Part model, mm, in its own coordinate system. Round coordinates to 2 decimals unless told otherwise and drop trailing zeros. Loops run counter-clockwise (first coordinate to the right, second up) from the corner with the lowest first, then second, coordinate; pieces in that order, holes last.
1) Band-saw the part on C-C, the plane z = 75. Write the cut outline in (x, y).
2) Band-saw the part on B-B, the plane x = -38.5. Write the cut outline in (y, z).
3) Band-saw the part on D-D, the plane x = -32. State how many separate pieces and enclosed holes the cut face has, then the cut area to 3 significant figures.
4) Band-saw the part on A-A, the plane z = 65. Write the cut outline in (x, y).
5) Probe line 1 (Y direction, x = -36.25, z = 65); line 2 (Z direction, x = -35, y = 7); line 3 (Z direction, x = -34.75, y = -10.5). List the from-to ranges inside material, lowest first.
6) Drop flat-ended pins along their axis: P1, Ø4.5, axis at y = -10, z = 65, coming from the -X side; P2, Ø3.5, axis at y = 0, z = 109, coming from the -X side; P3, Ø1.7, axis at y = 11, z = 125.5, coming from the +X side. Give the stop position or say it passes through.
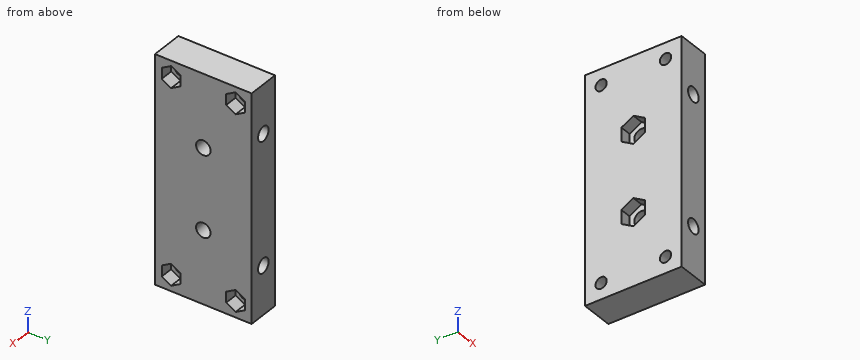
from build123d import *

# Parameters (mm, degrees)
SKETCH086_W     = 10
SKETCH086_H     = 70
SKETCH086_R     = 2.25
PAD058_DEPTH    = 15
SKETCH087_R     = 2.25
SKETCH087_R_2   = 1.75
POCKET021_DEPTH = 25
POCKET065_DEPTH = 3.5
POCKET066_DEPTH = 4


with BuildPart() as part:
    # Sketch086 → Pad058 (new body, symmetric)
    with BuildSketch(Plane.XZ):
        with Locations((-0.018685, 5)):
            Rectangle(SKETCH086_W, SKETCH086_H)
        with Locations((-0.018685, 25)):
            Circle(SKETCH086_R, mode=Mode.SUBTRACT)
        with Locations((-0.018685, -15)):
            Circle(SKETCH086_R, mode=Mode.SUBTRACT)
    extrude(amount=PAD058_DEPTH, both=True)

    # Sketch087 (on Face4 of Pad058) → Pocket021 (cut)
    with BuildSketch(Plane(origin=(-5.018685, 0, 0), x_dir=(0, 0, -1), z_dir=(-1, 0, 0))):
        with Locations((-17.5, 0)):
            Circle(SKETCH087_R)
        with Locations((7.5, 0)):
            Circle(SKETCH087_R)
        with Locations((-35, 10)):
            Circle(SKETCH087_R_2)
        with Locations((-35, -10)):
            Circle(SKETCH087_R_2)
        with Locations((25, 10)):
            Circle(SKETCH087_R_2)
        with Locations((25, -10)):
            Circle(SKETCH087_R_2)
    extrude(amount=-POCKET021_DEPTH, mode=Mode.SUBTRACT)

    # Sketch261 (on Face2 of Pocket021) → Pocket065 (cut)
    with BuildSketch(Plane(origin=(-5.018685, 0, 0), x_dir=(0, 0, -1), z_dir=(-1, 0, 0))):
        Polygon((-15.363804, 3.7), (-19.636196, 3.7), (-21.772392, 0), (-19.636196, -3.7), (-15.363804, -3.7), (-13.227608, 0), align=None)
        Polygon((9.636196, 3.7), (5.363804, 3.7), (3.227608, 0), (5.363804, -3.7), (9.636196, -3.7), (11.772392, 0), align=None)
    extrude(amount=-POCKET065_DEPTH, mode=Mode.SUBTRACT)

    # Sketch262 (on Face3 of Pocket065) → Pocket066 (cut)
    with BuildSketch(Plane(origin=(4.981315, 0, 0), x_dir=(0, 0, 1), z_dir=(1, 0, 0))):
        Polygon((36.674316, 12.9), (33.325684, 12.9), (31.651368, 10), (33.325684, 7.1), (36.674316, 7.1), (38.348632, 10), align=None)
        Polygon((36.674316, -7.1), (33.325684, -7.1), (31.651368, -10), (33.325684, -12.9), (36.674316, -12.9), (38.348632, -10), align=None)
        Polygon((-23.325684, -7.1), (-26.674316, -7.1), (-28.348632, -10), (-26.674316, -12.9), (-23.325684, -12.9), (-21.651368, -10), align=None)
        Polygon((-21.651368, 10), (-23.325684, 12.9), (-26.674316, 12.9), (-28.348632, 10), (-26.674316, 7.1), (-23.325684, 7.1), align=None)
    extrude(amount=-POCKET066_DEPTH, mode=Mode.SUBTRACT)


with BuildPart() as part_1:
    # Body043 placement: moved
    add(part.part.moved(Location((-35, 0, 90))))


solid = part_1.part
Reported:
1. outline: (-40.02, -15) - (-37.27, -15) - (-37.27, 15) - (-40.02, 15) - close; (-32.77, -15) - (-30.02, -15) - (-30.02, 15) - (-32.77, 15) - close
2. outline: (-15, 60) - (15, 60) - (15, 130) - (-15, 130) - close; hole circle Ø3.5 at (-10, 65); hole circle Ø3.5 at (-10, 125); hole (-3.7, 80.36) - (0, 78.23) - (3.7, 80.36) - (3.7, 84.64) - (0, 86.77) - (-3.7, 84.64) - close; hole (-3.7, 105.36) - (0, 103.23) - (3.7, 105.36) - (3.7, 109.64) - (0, 111.77) - (-3.7, 109.64) - close; hole circle Ø3.5 at (10, 65); hole circle Ø3.5 at (10, 125)
3. separate pieces: 1
3. enclosed holes: 6
3. area: 1,950 mm2
4. outline: (-40.02, -15) - (-30.02, -15) - (-30.02, -12.9) - (-34.02, -12.9) - (-34.02, -11.75) - (-40.02, -11.75) - close; (-40.02, -8.25) - (-34.02, -8.25) - (-34.02, -7.1) - (-30.02, -7.1) - (-30.02, 7.1) - (-34.02, 7.1) - (-34.02, 8.25) - (-40.02, 8.25) - close; (-40.02, 11.75) - (-34.02, 11.75) - (-34.02, 12.9) - (-30.02, 12.9) - (-30.02, 15) - (-40.02, 15) - close
5. line 1: y = -15 to -11.75, -8.25 to 8.25, 11.75 to 15
5. line 2: z = 60 to 72.75, 77.25 to 112.75, 117.25 to 130
5. line 3: z = 60 to 63.32, 66.68 to 72.77, 77.23 to 112.77, 117.23 to 123.32, 126.68 to 130
6. P1: stops at x = -40.02
6. P2: stops at x = -36.52
6. P3: stops at x = -34.02
